Here's how the part is built. I have some questions about the finished solid (model axes, mm). Round coordinates to 2 decimals unless told otherwise and drop trailing zeros. Order: outer loops, then holes, each group sorted by start corner. A loop starts at its lowest first (then second) coordinate and runs counter-clockwise, first axis right, second up.
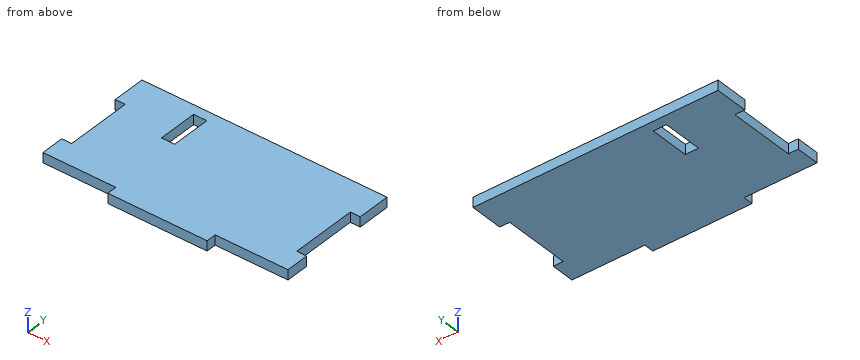
```python
from build123d import *

# Parameters (mm, degrees)
ESBO_O1_W                = 74
ESBO_O1_H                = 40
RESSALTO_EXTRUS_O1_DEPTH = 3
ESBO_O2_W                = 22
ESBO_O2_H                = 3
ESBO_O2_W_2              = 3
ESBO_O2_H_2              = 20
CORTE_EXTRUS_O1_DEPTH    = 3
ESBO_O3_W                = 4
ESBO_O3_H                = 12
CORTE_EXTRUS_O2_DEPTH    = 10


with BuildPart() as part:
    # Esboço1 → Ressalto-extrusão1 (new body)
    with BuildSketch(Plane.XY):
        Rectangle(ESBO_O1_W, ESBO_O1_H)
    extrude(amount=RESSALTO_EXTRUS_O1_DEPTH)

    # Esboço2 → Corte-extrusão1 (cut)
    with BuildSketch(Plane.XY.offset(3)):
        with Locations((-26, -18.5)):
            Rectangle(ESBO_O2_W, ESBO_O2_H)
        with Locations((26, -18.5)):
            Rectangle(ESBO_O2_W, ESBO_O2_H)
        with Locations((-35.5, 0)):
            Rectangle(ESBO_O2_W_2, ESBO_O2_H_2)
        with Locations((35.5, 0)):
            Rectangle(ESBO_O2_W_2, ESBO_O2_H_2)
    extrude(amount=-CORTE_EXTRUS_O1_DEPTH, mode=Mode.SUBTRACT)

    # Esboço3 → Corte-extrusão2 (cut)
    with BuildSketch(Plane.XY.offset(3)):
        with Locations((-17, 11)):
            Rectangle(ESBO_O3_W, ESBO_O3_H)
    extrude(amount=-CORTE_EXTRUS_O2_DEPTH, mode=Mode.SUBTRACT)


solid = part.part
```
1. I'm going to push flat-ended pins straight in: P1, Ø0.9, axis at y = 8.5, z = 1.5, coming from the +X side; P2, Ø0.9, axis at y = 5, z = 1, coming from the -X side; P3, Ø0.9, axis at x = -36, z = 1.5, coming from the -Y side; P4, Ø12, axis at x = -18, y = -14.5, coming from the -Z side. Where does each tip first touch, or does it pass through?
Evaluation:
P1: stops at x = 34
P2: stops at x = -34
P3: stops at y = -17
P4: stops at z = 0
2. If we section it at D-D, the plane y = -2.5: Write out the boundary of the cut face in (x, z), and give its area (3 significant figures).
Evaluation:
outline: (-34, 0) - (34, 0) - (34, 3) - (-34, 3) - close
area: 204 mm2
3. If we section it at B-B, the plane z = 0.55: Write out the boundary of the cut face in (x, y), and give its area (3 significant figures).
Evaluation:
outline: (-37, -17) - (-15, -17) - (-15, -20) - (15, -20) - (15, -17) - (37, -17) - (37, -10) - (34, -10) - (34, 10) - (37, 10) - (37, 20) - (-37, 20) - (-37, 10) - (-34, 10) - (-34, -10) - (-37, -10) - close; hole (-19, 5) - (-15, 5) - (-15, 17) - (-19, 17) - close
area: 2,660 mm2
4. If we section it at A-A, the plane y = 6.5: Write out the boundary of the cut face in (x, z).
Evaluation:
outline: (-34, 0) - (-19, 0) - (-19, 3) - (-34, 3) - close; (-15, 0) - (34, 0) - (34, 3) - (-15, 3) - close
5. I need wall thicknesses on probe 1 along X at (y, z) = (13, 2.2); probe 2 along Y at (x, z) = (-23.5, 1.1); probe 3 along X at (y, z) = (4.5, 1.8). Which ranges of each line are inside material? Lowest first, please.
Evaluation:
probe 1: x = -37 to -19, -15 to 37
probe 2: y = -17 to 20
probe 3: x = -34 to 34
6. If we section it at C-C, the plane x = -25: Write out the boundary of the cut face in (y, z), and give its area (3 significant figures).
Evaluation:
outline: (-17, 0) - (20, 0) - (20, 3) - (-17, 3) - close
area: 111 mm2
